from build123d import *

# Parameters (mm, degrees)
EXTRUDE_350_DEPTH = 5


with BuildPart() as part:
    # Эскиз2 → Extrude 350 (new body)
    with BuildSketch(Plane.XY):
        Polygon((5.773502692, 0), (2.886751346, 5), (-2.886751346, 5), (-5.773502692, 0), (-2.886751346, -5), (2.886751346, -5), align=None)
    extrude(amount=EXTRUDE_350_DEPTH)

    # Эскиз3 → Вырез-Повернуть1 (revolve, cut)
    with BuildSketch(Plane(origin=(0, 0, 0), x_dir=(1, 0, 0), z_dir=(0, 1, 0))):
        Polygon((-5.773502692, 0), (-4.5, 0), (-5.773502692, -0.735257122), align=None)
        Polygon((-5.773502692, -5), (-5.773502692, -4.264742878), (-4.5, -5), align=None)
    revolve(axis=Axis((0, 0, -10), (0, 0, 1)), mode=Mode.SUBTRACT)

    # Эскиз4 → Hole Wizard 701 (revolve, cut)
    with BuildSketch(Plane.YZ):
        Polygon((0, 0), (0, 5), (3, 5), (2.46, 4.46), (2.46, 0.54), (3, 0), align=None)
    revolve(axis=Axis((0, 0, -6.35), (0, 0, 1)), mode=Mode.SUBTRACT)


solid = part.part
Part model, mm, in its own coordinate system. Round coordinates to 2 decimals unless told otherwise and drop trailing zeros. Write each loop counter-clockwise with the first axis right and the second up, starting at its lowest first coordinate (ties: lowest second). Pieces come first, ordered by that corner, then holes. Notation, with made-up numbers: M -22,48 L 19,48 A9 ccw 19,53 Z; hole C 78.5,7.25 d5. An arc over 180 degrees is marked long. Return JSON: item names as keys, results as strings. Group by question number.
(1) Two-plate mould, pull along Y, no slides. Class faces 1 (the face through (4.31, -2.535, 2.469)), 2 (the face through (1, -3, 5)), 3 (the face through (0.942, 2.272, 2.473)), 4 (the face through (0, 5, 2)): +Y half, -Y half, draft (parallel to the pull), parting line (faces both ways), or undercut.
(2) Saw through at A-A on z = 3.85. Write the cut outline in (x, y).
(3) Pin check, flat tip, straight feed: pin 1 Ø1 at (x, y) = (-4.5, -3) entering from -Z. Stop position of the tip, or through.
(4) Saw through at B-B on x = 0. Write the cut outline in (y, z).
(5) Drill centre lines: probe 1 along Y at (x, z) = (0, 1.4); probe 2 along X at (y, z) = (1.75, 1.2); probe 3 along Y at (x, z) = (-2, 0.7). Where is each one in solid material? Low to high.
Returned:
{
 "1": {"face 1": "-Y half", "face 2": "draft", "face 3": "undercut", "face 4": "+Y half"},
 "2": {"outline": "M -5.77,0 L -2.89,-5 L 2.89,-5 L 5.77,0 L 2.89,5 L -2.89,5 Z; hole C 0,0 d4.92"},
 "3": {"pin 1": "z = 0.24"},
 "4": {"outline": "M -5,0.29 L -4.5,0 L -3,0 L -2.46,0.54 L -2.46,4.46 L -3,5 L -4.5,5 L -5,4.71 Z; M 2.46,0.54 L 3,0 L 4.5,0 L 5,0.29 L 5,4.71 L 4.5,5 L 3,5 L 2.46,4.46 Z"},
 "5": {"probe 1": "-5 to -2.46, 2.46 to 5", "probe 2": "-4.76 to -1.73, 1.73 to 4.76", "probe 3": "-5 to -1.43, 1.43 to 5"}
}
